from build123d import *

# Parameters (mm, degrees)
SALIENTE_EXTRUIR1_DEPTH              = 482
VACIADO1_T                           = -10
REDONDEO1_R                          = 10
REDONDEO2_R                          = 10
SALIENTE_EXTRUIR2_START              = -482
SALIENTE_EXTRUIR2_DEPTH              = 482
REDONDEO3_R                          = 5
SALIENTE_EXTRUIR3_DEPTH              = 10
SALIENTE_EXTRUIR4_DEPTH              = 10.2
SALIENTE_EXTRUIR5_START              = -10
SALIENTE_EXTRUIR5_DEPTH              = 10
RANURA_DE_MARGEN_PARA_M81_AT_2_COUNT = 2
RANURA_DE_MARGEN_PARA_M81_AT_2_PITCH = 83
RANURA_DE_MARGEN_PARA_M81_AT_3_COUNT = 2
RANURA_DE_MARGEN_PARA_M81_AT_3_PITCH = 166
RANURA_DE_MARGEN_PARA_M81_AT_4_COUNT = 2
RANURA_DE_MARGEN_PARA_M81_AT_4_PITCH = 249
RANURA_DE_MARGEN_PARA_M81_AT_5_COUNT = 2
RANURA_DE_MARGEN_PARA_M81_AT_5_PITCH = 332
RANURA_DE_MARGEN_PARA_M81_AT_6_COUNT = 2
RANURA_DE_MARGEN_PARA_M81_AT_6_PITCH = 415


with BuildPart() as part:
    # Croquis1 → Saliente-Extruir1 (new body)
    with BuildSketch(Plane.XY):
        with BuildLine():
            Line((0, 0), (230, 0))
            ThreePointArc((230, 0), (214.777511796, -36.557011873), (188.317948474, -66.019373845))
            ThreePointArc((188.317948474, -66.019373845), (182.470809449, -69.235256105), (175.891177547, -70.348529442))
            Line((175.891177547, -70.348529442), (54.108822453, -70.348529442))
            ThreePointArc((54.108822453, -70.348529442), (47.529190551, -69.235256105), (41.682051526, -66.019373845))
            ThreePointArc((41.682051526, -66.019373845), (15.222488204, -36.557011873), (0, 0))
        make_face()
    extrude(amount=SALIENTE_EXTRUIR1_DEPTH)

    # Vaciado1
    vaciado1_openings = [part.faces().sort_by_distance(p)[0] for p in [
        (115, 0, 241),
    ]]
    offset(amount=VACIADO1_T, openings=vaciado1_openings, kind=Kind.INTERSECTION)

    # Redondeo1
    redondeo1_edges = [part.edges().sort_by_distance(p)[0] for p in [
        (24.298628648, -32.189552634, 472),
        (50.819006502, -59.791892774, 472),
        (115, -60.348529442, 472),
        (179.180993498, -59.791892774, 472),
        (205.701371352, -32.189552634, 472),
    ]]
    fillet(redondeo1_edges, radius=REDONDEO1_R)

    # Redondeo2
    redondeo2_edges = [part.edges().sort_by_distance(p)[0] for p in [
        (24.298628648, -32.189552634, 10),
        (50.819006502, -59.791892774, 10),
        (115, -60.348529442, 10),
        (179.180993498, -59.791892774, 10),
        (205.701371352, -32.189552634, 10),
    ]]
    fillet(redondeo2_edges, radius=REDONDEO2_R)

    # Croquis2 → Saliente-Extruir2 (add)
    with BuildSketch(Plane.XY.offset(482).offset(SALIENTE_EXTRUIR2_START)):
        with BuildLine():
            Line((2.767082202, -10), (-25.0029178, -10))
            Line((-25.0029178, -10), (-25.0029178, 0))
            Line((-25.0029178, 0), (0, 0))
            ThreePointArc((0, 0), (1.273575047, -5.030428511), (2.767082202, -10))
        make_face()
        with BuildLine():
            Line((255.0029178, 0), (230, 0))
            ThreePointArc((230, 0), (228.726424953, -5.030428511), (227.232917798, -10))
            Line((227.232917798, -10), (255.0029178, -10))
            Line((255.0029178, -10), (255.0029178, 0))
        make_face()
    extrude(amount=SALIENTE_EXTRUIR2_DEPTH)

    # Redondeo3
    redondeo3_edges = [part.edges().sort_by_distance(p)[0] for p in [
        (-25.0029178, -10, 241),
        (255.0029178, -10, 241),
    ]]
    fillet(redondeo3_edges, radius=REDONDEO3_R)



with BuildPart() as body_2:
    # Croquis3 → Saliente-Extruir3 (new body)
    with BuildSketch(Plane(origin=(0, 0, 0), x_dir=(-1, 0, 0), z_dir=(0, 0, -1))):
        with BuildLine():
            Line((-10.515, 0), (-219.485, 0))
            ThreePointArc((-219.485, 0), (-188.589303813, 35.043815425), (-146.718891775, 55.767754196))
            ThreePointArc((-146.718891775, 55.767754196), (-115, 28), (-83.281108225, 55.767754196))
            ThreePointArc((-83.281108225, 55.767754196), (-41.410696187, 35.043815425), (-10.515, 0))
        make_face()
    extrude(amount=-SALIENTE_EXTRUIR3_DEPTH)


with BuildPart() as part_1:
    add(part.part)

    add(body_2.part)  # Saliente-Extruir4 merges body 2
    # Croquis4 → Saliente-Extruir4 (add)
    with BuildSketch(Plane(origin=(0, 0, 0), x_dir=(-1, 0, 0), z_dir=(0, 0, -1))):
        with BuildLine():
            ThreePointArc((-173.125860697, 45.121010845), (-115, 0), (-56.874139303, 45.121010845))
            ThreePointArc((-56.874139303, 45.121010845), (-69.763309442, 51.223971947), (-83.281108225, 55.767754196))
            ThreePointArc((-83.281108225, 55.767754196), (-115, 28), (-146.718891775, 55.767754196))
            ThreePointArc((-146.718891775, 55.767754196), (-160.236690558, 51.223971947), (-173.125860697, 45.121010845))
        make_face()
    extrude(amount=SALIENTE_EXTRUIR4_DEPTH)

    # Croquis5 → Saliente-Extruir5 (add)
    with BuildSketch(Plane.XY.offset(482).offset(SALIENTE_EXTRUIR5_START)):
        with BuildLine():
            ThreePointArc((83.281108225, 55.767754196), (41.410696187, 35.043815425), (10.515, 0))
            Line((10.515, 0), (219.485, 0))
            ThreePointArc((219.485, 0), (188.589303813, 35.043815425), (146.718891775, 55.767754196))
            ThreePointArc((146.718891775, 55.767754196), (115, 28), (83.281108225, 55.767754196))
        make_face()
        with BuildLine():
            ThreePointArc((90.133812203, 57.416842161), (86.69544771, 56.642215547), (83.281108225, 55.767754196))
            ThreePointArc((83.281108225, 55.767754196), (115, 28), (146.718891775, 55.767754196))
            ThreePointArc((146.718891775, 55.767754196), (143.30455229, 56.642215547), (139.866187797, 57.416842161))
            ThreePointArc((139.866187797, 57.416842161), (115, 35), (90.133812203, 57.416842161))
        make_face()
    extrude(amount=SALIENTE_EXTRUIR5_DEPTH)

    # Croquis8 → Ranura de margen para M81 (revolve, cut)
    with BuildSketch(Plane(origin=(-11.6229178, 0, 30), x_dir=(0, 0, 1), z_dir=(1, 0, 0))):
        Polygon((0, 0), (0, 92.5236146), (4.2, 90), (4.2, 0), align=None)
    ranura_de_margen_para_m81 = revolve(axis=Axis((-11.6229178, 6.35, 30), (0, -1, 0)), mode=Mode.SUBTRACT)

    # Ranura de margen para M81 at 2: Ranura de margen para M81 ×2
    with Locations(*[(0, 0, i * RANURA_DE_MARGEN_PARA_M81_AT_2_PITCH) for i in range(1, RANURA_DE_MARGEN_PARA_M81_AT_2_COUNT)]):
        add(ranura_de_margen_para_m81, mode=Mode.SUBTRACT)

    # Ranura de margen para M81 at 3: Ranura de margen para M81 ×2
    with Locations(*[(0, 0, i * RANURA_DE_MARGEN_PARA_M81_AT_3_PITCH) for i in range(1, RANURA_DE_MARGEN_PARA_M81_AT_3_COUNT)]):
        add(ranura_de_margen_para_m81, mode=Mode.SUBTRACT)

    # Ranura de margen para M81 at 4: Ranura de margen para M81 ×2
    with Locations(*[(0, 0, i * RANURA_DE_MARGEN_PARA_M81_AT_4_PITCH) for i in range(1, RANURA_DE_MARGEN_PARA_M81_AT_4_COUNT)]):
        add(ranura_de_margen_para_m81, mode=Mode.SUBTRACT)

    # Ranura de margen para M81 at 5: Ranura de margen para M81 ×2
    with Locations(*[(0, 0, i * RANURA_DE_MARGEN_PARA_M81_AT_5_PITCH) for i in range(1, RANURA_DE_MARGEN_PARA_M81_AT_5_COUNT)]):
        add(ranura_de_margen_para_m81, mode=Mode.SUBTRACT)

    # Ranura de margen para M81 at 6: Ranura de margen para M81 ×2
    with Locations(*[(0, 0, i * RANURA_DE_MARGEN_PARA_M81_AT_6_PITCH) for i in range(1, RANURA_DE_MARGEN_PARA_M81_AT_6_COUNT)]):
        add(ranura_de_margen_para_m81, mode=Mode.SUBTRACT)

    # Simetría1: Ranura de margen para M81 across plane
    add(ranura_de_margen_para_m81.mirror(Plane(origin=(115, 0, 0), x_dir=(0, 0, 1), z_dir=(1, 0, 0))), mode=Mode.SUBTRACT)

    # Simetría1 copy 1 sketch → Simetría1 copy 1 (revolve, cut)
    with BuildSketch(Plane(origin=(241.6229178, 0, 113), x_dir=(0, 0, 1), z_dir=(-1, 0, 0))):
        Polygon((0, 0), (0, -92.5236146), (4.2, -90), (4.2, 0), align=None)
    revolve(axis=Axis((241.6229178, 6.35, 113), (0, 1, 0)), mode=Mode.SUBTRACT)

    # Simetría1 copy 2 sketch → Simetría1 copy 2 (revolve, cut)
    with BuildSketch(Plane(origin=(241.6229178, 0, 196), x_dir=(0, 0, 1), z_dir=(-1, 0, 0))):
        Polygon((0, 0), (0, -92.5236146), (4.2, -90), (4.2, 0), align=None)
    revolve(axis=Axis((241.6229178, 6.35, 196), (0, 1, 0)), mode=Mode.SUBTRACT)

    # Simetría1 copy 3 sketch → Simetría1 copy 3 (revolve, cut)
    with BuildSketch(Plane(origin=(241.6229178, 0, 279), x_dir=(0, 0, 1), z_dir=(-1, 0, 0))):
        Polygon((0, 0), (0, -92.5236146), (4.2, -90), (4.2, 0), align=None)
    revolve(axis=Axis((241.6229178, 6.35, 279), (0, 1, 0)), mode=Mode.SUBTRACT)

    # Simetría1 copy 4 sketch → Simetría1 copy 4 (revolve, cut)
    with BuildSketch(Plane(origin=(241.6229178, 0, 362), x_dir=(0, 0, 1), z_dir=(-1, 0, 0))):
        Polygon((0, 0), (0, -92.5236146), (4.2, -90), (4.2, 0), align=None)
    revolve(axis=Axis((241.6229178, 6.35, 362), (0, 1, 0)), mode=Mode.SUBTRACT)

    # Simetría1 copy 5 sketch → Simetría1 copy 5 (revolve, cut)
    with BuildSketch(Plane(origin=(241.6229178, 0, 445), x_dir=(0, 0, 1), z_dir=(-1, 0, 0))):
        Polygon((0, 0), (0, -92.5236146), (4.2, -90), (4.2, 0), align=None)
    revolve(axis=Axis((241.6229178, 6.35, 445), (0, 1, 0)), mode=Mode.SUBTRACT)


solid = part_1.part
Design review of the part built by this model. Coordinates are the model's own, in mm. A direction names the side the tool comes from. Coordinates: 2 decimals unless noted, no trailing zeros. Order: outer loops, then holes, each group sorted by start corner. A loop starts at its lowest first (then second) coordinate and runs counter-clockwise, first axis right, second up. Notation, with made-up numbers: M -14.75,72 L -10.75,72 A25 cw -10.75,109 Z; hole C 84,13 d4. An arc over 180 degrees is marked long. Use a Markdown table: item, result.
(1) Add section B-B (z = 229). Give the boundary of the cut face in (x, y).
Worked answers:
| item | result |
|---|---|
| outline | M -25,-5 A5 ccw -20,-10 L 2.77,-10 A118 ccw 41.68,-66.02 A20 ccw 54.11,-70.35 L 175.89,-70.35 A20 ccw 188.32,-66.02 A118 ccw 227.23,-10 L 250,-10 A5 ccw 255,-5 L 255,0 L 219.71,0 A108 cw 182.1,-58.18 A10 cw 175.89,-60.35 L 54.11,-60.35 A10 cw 47.9,-58.18 A108 cw 10.29,0 L -25,0 Z |
(2) Draft analysis for pull direction Z (two halves, no side actions). For faces 4 (the cylindrical face through (212.19, -40.48, 237.63)), 5 (the flat face through (114, -8, 10)), 6 (the flat face through (113, -6, 482)), 7 (the flat face through (113, -25, 0)), state which applies: released by +Z, released by -Z, zero draft, split by the parting line, or undercut.
Worked answers:
| item | result |
|---|---|
| face 4 | zero draft |
| face 5 | undercut |
| face 6 | released by +Z |
| face 7 | released by -Z |
(3) For faces 1 (the cylindrical face through (116.11, 0.01, -5.03)), 2 (the cylindrical face through (114.15, -57.5, 13.01)), 3 (the cylindrical face through (114.356, 28.006, 0.041)), list the 3-axis set-ups (+Z, -Z, +X, -X, +Y, -Y) from which the entire face can be reached by the end or side of a thin tool; tool diameter is ignored.
Worked answers:
| item | result |
|---|---|
| face 1 | -Z, -Y |
| face 2 | +Y |
| face 3 | -Z, +Y |
(4) For P1, Ø9.5, axis at x = -11.62, z = 113, coming from the -Y side; P2, Ø13.5, axis at x = 241.62, z = 362, coming from the +Y side; P3, Ø8, axis at x = 91.5, y = -35, coming from the -Z side, all flat-tipped, find the tip position at first contact; note any pin that passes through.
Worked answers:
| item | result |
|---|---|
| P1 | stops at y = -10 |
| P2 | stops at y = 0 |
| P3 | stops at z = 0 |
(5) Add section A-A (y = 19). Give the boundary of the cut face in (x, z), then the cut area to 3 significant figures.
Worked answers:
| item | result |
|---|---|
| outline | M 24.23,0 L 71.19,0 L 71.19,-10.2 L 158.81,-10.2 L 158.81,0 L 205.77,0 L 205.77,10 L 24.23,10 Z; M 24.23,472 L 205.77,472 L 205.77,482 L 24.23,482 Z |
| area | 4,520 mm2 |
(6) Wall thickness on probe 1 along Z at (x, y) = (201, 22); probe 2 along Z at (x, y) = (146, 17.5); probe 3 along X at (y, z) = (-4.25, 113): over which ranges is each line inside the solid? List them lowest first.
Worked answers:
| item | result |
|---|---|
| probe 1 | z = 0 to 10, 472 to 482 |
| probe 2 | z = -10.2 to 10, 472 to 482 |
| probe 3 | x = -25 to -15.82, -7.42 to 11.45, 218.55 to 237.42, 245.82 to 255 |
